from build123d import *

# Parameters (mm, degrees)
EXTRUDE_1_DEPTH     = 16
SKETCH_3_W          = 8
SKETCH_3_H          = 20
SKETCH_3_H_2        = 25
CUT_EXTRUDE_1_DEPTH = 105.820083953
SKETCH_4_R          = 3
SKETCH_4_R_2        = 6
CUT_EXTRUDE_2_DEPTH = 105.012018536
CUT_EXTRUDE_3_DEPTH = 105.820083953
SKETCH_6_R          = 3
CUT_EXTRUDE_4_DEPTH = 105.012018536
EXTRUDE_2_DEPTH     = 15
CUT_EXTRUDE_START   = -15
CUT_EXTRUDE_5_DEPTH = 15
FILLET_1_R          = 7.5
SKETCH_9_R          = 2.5
CUT_EXTRUDE_6_DEPTH = 106.102331087


with BuildPart() as part:
    # 草图2 → 凸台-拉伸1 (new body)
    with BuildSketch(Plane(origin=(0, 0, 0), x_dir=(0, 0, -1), z_dir=(1, 0, 0))):
        with BuildLine():
            Line((-95, -7.5), (95, -7.5))
            ThreePointArc((95, -7.5), (102.5, 0), (95, 7.5))
            Line((95, 7.5), (-95, 7.5))
            ThreePointArc((-95, 7.5), (-102.5, 0), (-95, -7.5))
        make_face()
    extrude(amount=EXTRUDE_1_DEPTH)

    # 草图3 → 切除-拉伸1 (cut, through all)
    with BuildSketch(Plane(origin=(0, 7.5, 0), x_dir=(1, 0, 0), z_dir=(0, 1, 0))):
        with Locations((8, -92.5)):
            Rectangle(SKETCH_3_W, SKETCH_3_H)
        with Locations((8, 90)):
            Rectangle(SKETCH_3_W, SKETCH_3_H_2)
    extrude(amount=-CUT_EXTRUDE_1_DEPTH, mode=Mode.SUBTRACT)

    # 草图4 → 切除-拉伸2 (cut, through all)
    with BuildSketch(Plane(origin=(16, 0, 0), x_dir=(0, 0, -1), z_dir=(1, 0, 0))):
        with Locations((-95, 0)):
            Circle(SKETCH_4_R)
        with Locations((95, 0)):
            Circle(SKETCH_4_R_2)
    extrude(amount=-CUT_EXTRUDE_2_DEPTH, mode=Mode.SUBTRACT)

    # 草图5 → 切除-拉伸3 (cut, through all)
    with BuildSketch(Plane.XZ.offset(7.5)):
        with BuildLine():
            Line((12, 65), (12, -65))
            ThreePointArc((12, -65), (8, -69), (4, -65))
            Line((4, -65), (4, 65))
            ThreePointArc((4, 65), (8, 69), (12, 65))
        make_face()
    extrude(amount=-CUT_EXTRUDE_3_DEPTH, mode=Mode.SUBTRACT)

    # 草图6 → 切除-拉伸4 (cut, through all)
    with BuildSketch(Plane.ZY):
        with Locations((15, 0)):
            Circle(SKETCH_6_R)
    extrude(amount=-CUT_EXTRUDE_4_DEPTH, mode=Mode.SUBTRACT)

    # 草图7 → 凸台-拉伸2 (add)
    with BuildSketch(Plane.XZ.offset(7.5)):
        with BuildLine():
            Line((7.022963208, -77.5), (0, -77.5))
            ThreePointArc((0, -77.5), (-0.707106781, -77.792893219), (-1, -78.5))
            Line((-1, -78.5), (-1, -102.5))
            Line((-1, -102.5), (-3, -102.5))
            Line((-3, -102.5), (-3, -73.5))
            ThreePointArc((-3, -73.5), (-2.707106781, -72.792893219), (-2, -72.5))
            Line((-2, -72.5), (0, -72.5))
            Line((0, -72.5), (0, -76.537771908))
            Line((0, -76.537771908), (16, -76.537771908))
            Line((16, -76.537771908), (16, -72.5))
            Line((16, -72.5), (18, -72.5))
            ThreePointArc((18, -72.5), (18.707106781, -72.792893219), (19, -73.5))
            Line((19, -73.5), (19, -102.5))
            Line((19, -102.5), (17, -102.5))
            Line((17, -102.5), (17, -78.5))
            ThreePointArc((17, -78.5), (16.707106781, -77.792893219), (16, -77.5))
            Line((16, -77.5), (8.977036792, -77.5))
            Line((8.977036792, -77.5), (7.022963208, -77.5))
        make_face()
    extrude(amount=-EXTRUDE_2_DEPTH)

    # 草图8 → 切除-拉伸5 (cut)
    with BuildSketch(Plane(origin=(0, -7.5, 0), x_dir=(-1, 0, 0), z_dir=(0, -1, 0)).offset(CUT_EXTRUDE_START)):
        with BuildLine():
            Line((-17, 102.5), (1, 102.5))
            Line((1, 102.5), (1, 78.5))
            ThreePointArc((1, 78.5), (0.707106781, 77.792893219), (0, 77.5))
            Line((0, 77.5), (-16, 77.5))
            ThreePointArc((-16, 77.5), (-16.707106781, 77.792893219), (-17, 78.5))
            Line((-17, 78.5), (-17, 102.5))
        make_face()
    extrude(amount=CUT_EXTRUDE_5_DEPTH, mode=Mode.SUBTRACT)

    # 圆角1
    fillet_1_edges = [part.edges().sort_by_distance(p)[0] for p in [
        (18, 7.5, -102.5),
        (18, -7.5, -102.5),
        (-2, 7.5, -102.5),
        (-2, -7.5, -102.5),
    ]]
    fillet(fillet_1_edges, radius=FILLET_1_R - 0.0001)  # a hair under: the kernel refuses the full size

    # 草图9 → 切除-拉伸6 (cut, through all)
    with BuildSketch(Plane(origin=(19, 0, 0), x_dir=(0, 0, -1), z_dir=(1, 0, 0))):
        with Locations((95, 0)):
            Circle(SKETCH_9_R)
    extrude(amount=-CUT_EXTRUDE_6_DEPTH, mode=Mode.SUBTRACT)


solid = part.part
Work out the finished part from the listing and answer in its coordinate system (mm). A direction names the side the tool comes from. Round coordinates to 2 decimals unless told otherwise and drop trailing zeros. Loops run counter-clockwise (first coordinate to the right, second up) from the corner with the lowest first, then second, coordinate; pieces in that order, holes last. Notation, with made-up numbers: (0.25, -39) -> (55.25, -39) arc R22 ccw to (55.25, -1) -> close; hole circle Ø1 at (25, 33). An arc over 180 degrees is marked (long way). Use one line per item in the form item = value.
(1) Find section C-C on z = 50. Give the vertices of the cut face in (x, y), then the cut area to 3 significant figures.
Answer list:
outline = (0, -7.5) -> (4, -7.5) -> (4, 7.5) -> (0, 7.5) -> close; (12, -7.5) -> (16, -7.5) -> (16, 7.5) -> (12, 7.5) -> close
area = 120 mm2
(2) Flat-ended cylindrical pins translate along their axes: P1, Ø7, axis at y = 0, z = 95, coming from the -X side; P2, Ø1, axis at x = 17, y = 1, coming from the +Z side; P3, Ø7.5, axis at y = 3.5, z = -17.5, coming from the +X side; P4, Ø6.5, axis at y = 0, z = -95, coming from the -X side. Find the tip coordinate at first contact, or state that the pin passes through.
Answer list:
P1 = 0
P2 = -72.5
P3 = 16
P4 = -3
(3) Find section B-B on z = 15. Give the vertices of the cut face in (x, y).
Answer list:
outline = (0, -7.5) -> (4, -7.5) -> (4, -3) -> (0, -3) -> close; (0, 3) -> (4, 3) -> (4, 7.5) -> (0, 7.5) -> close; (12, -7.5) -> (16, -7.5) -> (16, -3) -> (12, -3) -> close; (12, 3) -> (16, 3) -> (16, 7.5) -> (12, 7.5) -> close
(4) A tool of negligible diameter and unlimited length cuts with its end or side. For faces 1 (the flat face through (12, 0, 90)), 2 (the flat face through (-1, 0, -90)), 3 (the flat face through (13, 7.5, 1)), 4 (the cylindrical face through (8, 0, -69)), 5 (the cylindrical face through (14, 0, 12)), from which of +Z, -Z, +X, -X, +Y, -Y can it reach the whole face along a straight path? Write none if from no direction.
Answer list:
face_1 = +Z, +Y, -Y
face_2 = -Z, +Y, -Y
face_3 = +Z, -Z, +X, -X, +Y
face_4 = +Y, -Y
face_5 = +X, -X
(5) Straight lines are drawn through the part: line 1 (Y direction, x = 2.7, z = 95); line 2 (Z direction, x = 2.25, y = 0.75); line 3 (X direction, y = -0.75, z = -47). For each, find the intervals that lie inside material, in ascending order.
Answer list:
line_1 = -7.5 to -3, 3 to 7.5
line_2 = -77.5 to 12.1, 17.9 to 92.1, 97.9 to 102.46
line_3 = 0 to 4, 12 to 16
(6) Find section A-A on x = 8. Give the vertices of the cut face in (y, z), then the cut area to 3 significant figures.
Answer list:
outline = (-7.5, -77.5) -> (7.5, -77.5) -> (7.5, -69) -> (-7.5, -69) -> close; (-7.5, 69) -> (7.5, 69) -> (7.5, 82.5) -> (-7.5, 82.5) -> close
area = 330 mm2
(7) For a pull along Z with two mould halves and no side action, classify faces 6 (the cylindrical face through (8, 0, 69)), 7 (the flat face through (8, 0, -77.5)), 8 (the flat face through (19, 0, -88)), 9 (the cylindrical face through (1.97, 0.16, 102.5)) as released by +Z, released by -Z, zero draft, split by the parting line, or undercut.
Answer list:
face_6 = undercut
face_7 = released by -Z
face_8 = zero draft
face_9 = released by +Z
